The model under review builds one solid part; all positions refer to its coordinate system, in mm. Face numbers are marked on the shaded views. A direction names the side the tool comes from. Coordinates: 2 decimals unless noted, no trailing zeros. Loops run counter-clockwise (first coordinate to the right, second up) from the corner with the lowest first, then second, coordinate; pieces in that order, holes last. Notation, with made-up numbers: (54, 67) - (60, 67) arc R14 cw to (60, 87) - close; hole circle Ø10 at (70, 5). An arc over 180 degrees is marked (long way). Answer in a Markdown table with one row per item. Add a question column.
(1) We need section C-C on x = 15. Write out the cut boundary in (y, z), plus the area to 4 significant figures.
(2) We need section B-B on y = 17.15. Write out the cut boundary in (x, z), plus the area to 3 significant figures.
(3) For line 1 along Y through (x, z) = (12.25, 7.5); line 2 along X through (y, z) = (15.7, 7.75); line 3 along Z through (x, y) = (16, 13.7), list the stretches that pass through material, from the lowest coordinate up.
(4) For P1, Ø0.5, axis at x = 18.5, y = 17, coming from the -Z side; P2, Ø0.5, axis at x = 11.5, z = 8, coming from the -Y side; P3, Ø0.8, axis at x = 18.5, z = 7, coming from the +Y side, all flat-tipped, find the tip position at first contact; note any pin that passes through.
(5) Machinability: for the marked faces 5, 6 and 7, which of the approach directions +Z, -Z, +X, -X, +Y, -Y give a long, thin tool a straight path to every point of the face, cutting with its end or side? Answer none if there is none.
(6) We need section D-D on z = 15. Write out the cut boundary in (x, y), plus the area to 3 significant figures.
(7) Mouldability with a two-part tool opening along X and no side actions: class the marked faces 1, 2, 3 and 4 as +X half, -X half, draft (parallel to the pull), parting line (faces both ways), or undercut.
from build123d import *

# Parameters (mm, degrees)
BOX004_W       = 1
BOX004_H       = 3.5
BOX004_DEPTH   = 4
BOX005_W       = 1
BOX005_H       = 3.5
BOX005_DEPTH   = 4
CYLINDER_R     = 2
CYLINDER_DEPTH = 3
BOX006_W       = 6
BOX006_H       = 1
BOX006_DEPTH   = 4
BOX007_W       = 6
BOX007_H       = 1
BOX007_DEPTH   = 4
BOX003_W       = 8
BOX003_H       = 5.5
BOX003_DEPTH   = 4.5


with BuildPart() as cube001:
    # Box004 → Box004 (new body)
    with BuildSketch(Plane(origin=(11, 13, 5), x_dir=(1, 0, 0), z_dir=(0, 0, 1))):
        with Locations((0.5, 1.75)):
            Rectangle(BOX004_W, BOX004_H)
    extrude(amount=BOX004_DEPTH)


with BuildPart() as cube002:
    # Box005 → Box005 (new body)
    with BuildSketch(Plane(origin=(18, 13, 5), x_dir=(1, 0, 0), z_dir=(0, 0, 1))):
        with Locations((0.5, 1.75)):
            Rectangle(BOX005_W, BOX005_H)
    extrude(amount=BOX005_DEPTH)


with BuildPart() as cylinder:
    # Cylinder → Cylinder (new body)
    with BuildSketch(Plane(origin=(15, 14.75, 13), x_dir=(1, 0, 0), z_dir=(0, 0, 1))):
        Circle(CYLINDER_R)
    extrude(amount=CYLINDER_DEPTH)


with BuildPart() as cube003:
    # Box006 → Box006 (new body)
    with BuildSketch(Plane(origin=(12, 12, 5), x_dir=(1, 0, 0), z_dir=(0, 0, 1))):
        with Locations((3, 0.5)):
            Rectangle(BOX006_W, BOX006_H)
    extrude(amount=BOX006_DEPTH)


with BuildPart() as cube004:
    # Box007 → Box007 (new body)
    with BuildSketch(Plane(origin=(12, 16.5, 5), x_dir=(1, 0, 0), z_dir=(0, 0, 1))):
        with Locations((3, 0.5)):
            Rectangle(BOX007_W, BOX007_H)
    extrude(amount=BOX007_DEPTH)


with BuildPart() as bt_ex001:
    # Box003 → Box003 (new body)
    with BuildSketch(Plane(origin=(11, 12, 9), x_dir=(1, 0, 0), z_dir=(0, 0, 1))):
        with Locations((4, 2.75)):
            Rectangle(BOX003_W, BOX003_H)
    extrude(amount=BOX003_DEPTH)

    # Fusion: union Cube001, Cube002, Cylinder, Cube003, Cube004
    add(cube001.part)
    add(cube002.part)
    add(cylinder.part)
    add(cube003.part)
    add(cube004.part)


solid = bt_ex001.part
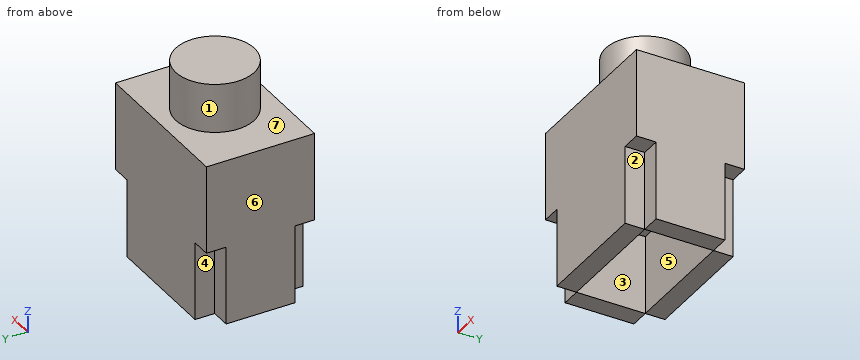
Outcome:
| question | item | result |
|---|---|---|
| 1 | outline | (12, 5) - (13, 5) - (13, 9) - (16.5, 9) - (16.5, 5) - (17.5, 5) - (17.5, 13.5) - (16.75, 13.5) - (16.75, 16) - (12.75, 16) - (12.75, 13.5) - (12, 13.5) - close |
| 1 | area | 42.75 mm² |
| 2 | outline | (11, 9) - (12, 9) - (12, 5) - (18, 5) - (18, 9) - (19, 9) - (19, 13.5) - (11, 13.5) - close |
| 2 | area | 60.0 mm² |
| 3 | line 1 | 12 to 13, 16.5 to 17.5 |
| 3 | line 2 | 11 to 12, 18 to 19 |
| 3 | line 3 | 9 to 16 |
| 4 | P1 | z = 9 |
| 4 | P2 | y = 13 |
| 4 | P3 | y = 16.5 |
| 5 | face 5 | -Z |
| 5 | face 6 | +Z, -Z, -X, +Y, -Y |
| 5 | face 7 | +Z |
| 6 | outline | circle Ø4 at (15, 14.75) |
| 6 | area | 12.6 mm² |
| 7 | face 1 | parting line |
| 7 | face 2 | +X half |
| 7 | face 3 | undercut |
| 7 | face 4 | -X half |
